from build123d import *

# Parameters (mm, degrees)
CROQUIS1_W              = 18
CROQUIS1_H              = 73.2
CROQUIS1_R              = 6.5
CROQUIS1_R_2            = 1
CROQUIS1_W_2            = 10
CROQUIS1_H_2            = 3.2
SALIENTE_EXTRUIR1_DEPTH = 3
REDONDEO1_R             = 5


with BuildPart() as part:
    # Croquis1 → Saliente-Extruir1 (new body)
    with BuildSketch(Plane(origin=(0, 0, 0), x_dir=(0, 0, -1), z_dir=(1, 0, 0))):
        Rectangle(CROQUIS1_W, CROQUIS1_H)
        with Locations((0, 20.1)):
            Circle(CROQUIS1_R, mode=Mode.SUBTRACT)
        with Locations(Location((0, -20.1, 0), (0, 0, 180))):
            Circle(CROQUIS1_R, mode=Mode.SUBTRACT)
        with Locations((-5, 0)):
            Circle(CROQUIS1_R_2, mode=Mode.SUBTRACT)
        with Locations(Location((5, 0, 0), (0, 0, 180))):
            Circle(CROQUIS1_R_2, mode=Mode.SUBTRACT)
        with Locations((0, -5)):
            Rectangle(CROQUIS1_W_2, CROQUIS1_H_2, mode=Mode.SUBTRACT)
    extrude(amount=SALIENTE_EXTRUIR1_DEPTH)

    # Redondeo1
    redondeo1_edges = [part.edges().sort_by_distance(p)[0] for p in [
        (1.5, 36.6, 9),
        (1.5, -36.6, 9),
    ]]
    fillet(redondeo1_edges, radius=REDONDEO1_R)


solid = part.part
Build history of the part. All positions in model axes, mm. A direction names the side the tool comes from. Round coordinates to 2 decimals unless told otherwise and drop trailing zeros. Write each loop counter-clockwise with the first axis right and the second up, starting at its lowest first coordinate (ties: lowest second). Pieces come first, ordered by that corner, then holes. Notation, with made-up numbers: M -9.75,85 L 29.25,85 A6 cw 29.25,96 Z; hole C 7.5,-29 d3. An arc over 180 degrees is marked long. Answer in a Markdown table with one row per item.
1. Saw through at B-B (y = -20.1). List the corners of the cut face in (x, z), and give its area (3 significant figures).
Geometry check:
| item | result |
|---|---|
| outline | M 0,-9 L 3,-9 L 3,-6.5 L 0,-6.5 Z; M 0,6.5 L 3,6.5 L 3,9 L 0,9 Z |
| area | 15.0 mm2 |
2. Saw through at A-A (z = 0). List the corners of the cut face in (x, y), and give its area (3 significant figures).
Geometry check:
| item | result |
|---|---|
| outline | M 0,-36.6 L 3,-36.6 L 3,-26.6 L 0,-26.6 Z; M 0,-13.6 L 3,-13.6 L 3,-6.6 L 0,-6.6 Z; M 0,-3.4 L 3,-3.4 L 3,13.6 L 0,13.6 Z; M 0,26.6 L 3,26.6 L 3,36.6 L 0,36.6 Z |
| area | 132 mm2 |
3. Mould opens along Y. For faces 3 (the face through (1.52, 35.1, 7.57)), 4 (the face through (3, 1, 0)), 5 (the face through (1, -5, 5)) say: +Y half, -Y half, draft (parallel to the pull), parting line (faces both ways), or undercut.
Geometry check:
| item | result |
|---|---|
| face 3 | +Y half |
| face 4 | draft |
| face 5 | undercut |
4. Saw through at D-D (x = 1.7). List the corners of the cut face in (y, z).
Geometry check:
| item | result |
|---|---|
| outline | M -36.6,-9 L 36.6,-9 L 36.6,4 A5 ccw 31.6,9 L -31.6,9 A5 ccw -36.6,4 Z; hole C -20.1,0 d13; hole M -6.6,-5 L -3.4,-5 L -3.4,5 L -6.6,5 Z; hole C 0,-5 d2; hole C 0,5 d2; hole C 20.1,0 d13 |
5. Saw through at C-C (y = 0). List the corners of the cut face in (x, z), and give its area (3 significant figures).
Geometry check:
| item | result |
|---|---|
| outline | M 0,-9 L 3,-9 L 3,-6 L 0,-6 Z; M 0,-4 L 3,-4 L 3,4 L 0,4 Z; M 0,6 L 3,6 L 3,9 L 0,9 Z |
| area | 42.0 mm2 |
6. Probe L1, parallel to Y at x = 1.85, z = 0; L2, parallel to Z at x = 0.3, y = -3.5; L3, parallel to Z at x = 2.25, y = -20.1. List the from-to ranges inside material, lowest first. Write a range as [from, to].
Geometry check:
| item | result |
|---|---|
| L1 | [-36.6, -26.6], [-13.6, -6.6], [-3.4, 13.6], [26.6, 36.6] |
| L2 | [-9, -5], [5, 9] |
| L3 | [-9, -6.5], [6.5, 9] |
7. Which spindle directions (+Z, -Z, +X, -X, +Y, -Y) get a long thin tool onto all of the face, cutting with end or side? Do faces 1 (the face through (1.52, -35.1, 7.57)), 2 (the face through (1, -6.6, 0)). Say none if no direction does.
Geometry check:
| item | result |
|---|---|
| face 1 | +Z, +X, -X, -Y |
| face 2 | +X, -X |
